For this review, take the finished solid that the model builds, in its own axes (mm). A direction names the side the tool comes from. Round coordinates to 2 decimals unless told otherwise and drop trailing zeros. Order: outer loops, then holes, each group sorted by start corner. A loop starts at its lowest first (then second) coordinate and runs counter-clockwise, first axis right, second up. Notation, with made-up numbers: (19, -23) -> (59, -23) arc R13 ccw to (59, -1) -> close; hole circle Ø3 at (30.25, -22). An arc over 180 degrees is marked (long way). Use a Markdown table: item, result. Add a question column.
1) Consider section B-B (x = 2.5). State the section outline as (y, z) points.
2) Draft analysis for pull direction X (two halves, no side actions). For faces 3 (the face through (2, -10, -30)), 4 (the face through (9.59, -0.32, 24.97)), 5 (the face through (4, -9, 3)), 6 (the face through (10.57, -15.2, 35.67)), state which applies: pulls with the +X half, pulls with the -X half, needs draft (parallel to the pull), parting line crosses it, or undercut.
3) Clearance check with flat-ended pins moving along their axes: P1, Ø6, axis at y = -1, z = 20, coming from the +X side; P2, Ø1.5, axis at x = 6, y = -4, coming from the -Z side; P3, Ø1.5, axis at x = 2, z = 8.5, coming from the +Y side; P4, Ø8, axis at x = 12, y = -11.5, coming from the +Z side. State where each tip first meets the part, or that it passes through.
4) Consider section C-C (y = -10). Give the number of separate pieces and of enclosed holes in the cut face, plus the area to 3 significant figures.
5) Machinability: for faces 1 (the face through (10.41, -7.64, 27.81)), 2 (the face through (8.381, -18.849, 38.298)), which of the approach directions +Z, -Z, +X, -X, +Y, -Y give a long, thin tool a straight path to every point of the face, cutting with its end or side? Answer none if there is none.
6) Consider section D-D (x = 13). State the section outline as (y, z) points.
7) Consider section A-A (z = 0). State the section outline as (x, y) points, plus the area to 3 significant figures.
8) Wall thickness on line 1 along Y through (x, z) = (2.15, -20); line 2 along X through (y, z) = (-9.25, 17.5); line 3 along Y through (x, z) = (3, 2): over which ranges is each line inside the solid? List them lowest first. Write a range as [from, to].
```python
from build123d import *

# Parameters (mm, degrees)
SKETCH1_W           = 40
SKETCH1_H           = 20
SKETCH1_R           = 2.78
BOSS_EXTRUDE1_DEPTH = 4
SKETCH6_W           = 17
SKETCH6_H           = 24.632994134
SKETCH6_R           = 1.5
BOSS_EXTRUDE2_DEPTH = 4


with BuildPart() as part:
    # Sketch1 → Boss-Extrude1 (new body)
    with BuildSketch(Plane(origin=(0, 0, 0), x_dir=(0, 0, -1), z_dir=(1, 0, 0))):
        with Locations((10, -10)):
            Rectangle(SKETCH1_W, SKETCH1_H)
        with Locations((0, -10)):
            Circle(SKETCH1_R, mode=Mode.SUBTRACT)
        with Locations((20, -10)):
            Circle(SKETCH1_R, mode=Mode.SUBTRACT)
    extrude(amount=BOSS_EXTRUDE1_DEPTH)

    # Sketch5 → section 0 of loft1
    with BuildSketch(Plane(origin=(0, 10.577438307, 14.711318924), x_dir=(1, 0, 0), z_dir=(0, 0.5837698787992286, 0.8119191638375918)), mode=Mode.PRIVATE) as loft1_s0:
        with BuildLine():
            Line((0, -13.027698788), (4, -13.027698788))
            Line((4, -13.027698788), (4, -37.660692922))
            Line((4, -37.660692922), (0, -37.660692922))
            Line((0, -37.660692922), (0, -13.027698788))
        make_face()
    # loft up to a face of the part (loft1)
    loft([loft1_s0.sketch, part.faces().sort_by_distance((2, -10, 10))[0]])

    # Sketch6 → Boss-Extrude2 (add)
    with BuildSketch(Plane(origin=(0, 10.577438307, 14.711318924), x_dir=(1, 0, 0), z_dir=(0, 0.5837698787992287, 0.8119191638375917))):
        with Locations((8.5, -25.344195855)):
            Rectangle(SKETCH6_W, SKETCH6_H)
        with Locations(Location((10.5, -20.500692922, 0), (0, 0, 270))):
            Circle(SKETCH6_R, mode=Mode.SUBTRACT)
        with Locations(Location((10.5, -25.580692922, 0), (0, 0, 270))):
            Circle(SKETCH6_R, mode=Mode.SUBTRACT)
        with Locations(Location((10.5, -30.660692922, 0), (0, 0, 270))):
            Circle(SKETCH6_R, mode=Mode.SUBTRACT)
        with Locations(Location((10.5, -34.660692922, 0), (0, 0, 270))):
            Circle(SKETCH6_R, mode=Mode.SUBTRACT)
        with Locations(Location((10.5, -16.027698788, 0), (0, 0, 270))):
            Circle(SKETCH6_R, mode=Mode.SUBTRACT)
    extrude(amount=BOSS_EXTRUDE2_DEPTH)


solid = part.part
```
Results list:
| question | item | result |
|---|---|---|
| 1 | outline | (-20, -30) -> (0, -30) -> (0, 22.32) -> (2.34, 25.56) -> (-17.66, 39.94) -> (-20, 36.7) -> close; hole circle Ø5.56 at (-10, -20); hole circle Ø5.56 at (-10, 0) |
| 2 | face 3 | needs draft |
| 2 | face 4 | undercut |
| 2 | face 5 | pulls with the +X half |
| 2 | face 6 | undercut |
| 3 | P1 | x = 17 |
| 3 | P2 | z = 24.65 |
| 3 | P3 | y = 0 |
| 3 | P4 | z = 38.39 |
| 4 | separate pieces | 3 |
| 4 | enclosed holes | 0 |
| 4 | area | 270 mm2 |
| 5 | face 1 | -Z, +X, -Y |
| 5 | face 2 | +Z, +X, -X, -Y |
| 6 | outline | (-20, 36.7) -> (0, 22.32) -> (2.34, 25.56) -> (-17.66, 39.94) -> close |
| 7 | outline | (0, -20) -> (4, -20) -> (4, -12.78) -> (0, -12.78) -> close; (0, -7.22) -> (4, -7.22) -> (4, 0) -> (0, 0) -> close |
| 7 | area | 57.8 mm2 |
| 8 | line 1 | [-20, -12.78], [-7.22, 0] |
| 8 | line 2 | [0, 4] |
| 8 | line 3 | [-20, -11.93], [-8.07, 0] |
